Work out the finished part from the listing and answer in its coordinate system (mm). A direction names the side the tool comes from. Round coordinates to 2 decimals unless told otherwise and drop trailing zeros. Order: outer loops, then holes, each group sorted by start corner. A loop starts at its lowest first (then second) coordinate and runs counter-clockwise, first axis right, second up. Notation, with made-up numbers: (-30, 27.25) -> (-23, 27.25) arc R30 cw to (-23, 60.25) -> close; hole circle Ø7 at (14, 4). An arc over 180 degrees is marked (long way). Use one line per item in the form item = value.
```python
from build123d import *

# Parameters (mm, degrees)
F1_DEPTH = 60
F3_DEPTH = 80
F4_W     = 6.1120763421
F4_H     = 50.4245881457
F5_DEPTH = 57.3
F7_DEPTH = 45.7
F8_R     = 30


with BuildPart() as f1:
    # F0 (on Right) → F1 (new body)
    with BuildSketch(Plane.YZ):
        Polygon((-85.0046053529, 28.4824129194), (-95.0890108943, 3.9917188697), (-95.0890108943, -38.8669967651), (43.5715354979, -38.8669967651), (54.0160946548, -6.812999025), (28.4449271858, 52.252791822), (-15.8544126898, 52.252791822), (-15.8544126898, 8.3136055619), (-23.7778741866, 28.4824129194), align=None)
    extrude(amount=F1_DEPTH)

    # F2 (on face) → F3 (join)
    with BuildSketch(Plane.YZ.offset(60)):
        Polygon((-9.2091018375, -8.6017280287), (-15.8544126898, 8.3136055619), (-23.7778741866, 28.4824129194), (-85.0046053529, 28.4824129194), (-95.0890108943, 3.9917188697), (-95.0890108943, -38.8669967651), (43.5715354979, -38.8669967651), (53.433250479, -8.6017280287), align=None)
    extrude(amount=F3_DEPTH)

    # F4 (on face) → F5 (join)
    with BuildSketch(Plane.XY.offset(-8.6017280287)):
        with Locations((78.1879983842, 23.0138575425)):
            Rectangle(F4_W, F4_H)
        with Locations((106.4563281834, 23.0138575425)):
            Rectangle(F4_W, F4_H)
    extrude(amount=F5_DEPTH)

    # F6 (on face) → F7 (cut)
    with BuildSketch(Plane.YZ.offset(109.5123663545)):
        Polygon((-2.1984365303, 48.6982719713), (-2.1984365303, 32.272413373), (24.9238815159, 32.272413373), (48.2261516154, 7.0601203479), (48.2261516154, 48.6982719713), align=None)
    extrude(amount=-F7_DEPTH, mode=Mode.SUBTRACT)

    # F8
    f8_edges = [f1.edges().sort_by_distance(p)[0] for p in [
        (106.456328, 48.226152, 7.06012),
        (106.456328, 24.923882, 32.272413),
        (78.187998, 24.923882, 32.272413),
        (78.187998, 48.226152, 7.06012),
    ]]
    fillet(f8_edges, radius=F8_R)


solid = f1.part
```
Item 1: The part is cut by section B-B, the plane x = 94. Give the vertices of the cut face in (y, z).
Findings:
outline = (-95.09, -38.87) -> (43.57, -38.87) -> (53.43, -8.6) -> (-9.21, -8.6) -> (-23.78, 28.48) -> (-85, 28.48) -> (-95.09, 3.99) -> close
Item 2: The part is cut by section A-A, the plane z = 18. Give the vertices of the cut face in (x, y).
Findings:
outline = (0, -89.32) -> (140, -89.32) -> (140, -19.66) -> (0, -19.66) -> close; (0, -15.85) -> (60, -15.85) -> (60, 43.27) -> (0, 43.27) -> close; (75.13, -2.2) -> (81.24, -2.2) -> (81.24, 38.12) -> (75.13, 38.12) -> close; (103.4, -2.2) -> (109.51, -2.2) -> (109.51, 38.12) -> (103.4, 38.12) -> close
Item 3: Consider line 1 along X through (y, z) = (18, 6); line 2 along Y through (x, z) = (13, 20.5); line 3 along Z through (x, y) = (109, 6). Determine where each line is inside the solid, lowest interval first.
Findings:
line_1 = 0 to 60, 75.13 to 81.24, 103.4 to 109.51
line_2 = -88.29 to -20.64, -15.85 to 42.19
line_3 = -38.87 to 32.27
Item 4: The part is cut by section C-C, the plane y = -59.5. Give the vertices of the cut face in (x, z), and give its area (3 significant figures).
Findings:
outline = (0, -38.87) -> (140, -38.87) -> (140, 28.48) -> (0, 28.48) -> close
area = 9,430 mm^2
Item 5: The part is cut by section D-D, the plane x = 55. Give the vertices of the cut face in (y, z), and give its area (3 significant figures).
Findings:
outline = (-95.09, -38.87) -> (43.57, -38.87) -> (54.02, -6.81) -> (28.44, 52.25) -> (-15.85, 52.25) -> (-15.85, 8.31) -> (-23.78, 28.48) -> (-85, 28.48) -> (-95.09, 3.99) -> close
area = 10,600 mm^2
Item 6: For faces 1 (the flat face through (106.499, 36.999, 19.207)), 2 (the flat face through (30, -15.854, 31)), 3 (the flat face through (69, -54, 28.482)), 4 (the flat face through (60, 11, 22)), 5 (the flat face through (106, 5, 32.272)), determine the directions among +Z, -Z, +X, -X, +Y, -Y from which every point of the face is accessible in a straight line to the end or side of a thin tool.
Findings:
face_1 = +Z, +X, +Y
face_2 = +Z, +X, -X
face_3 = +Z, +X, -X, -Y
face_4 = +Z, +Y
face_5 = +Z, +X, +Y, -Y
Item 7: Determine the mould class of faces 6 (the flat face through (106, -2.198, 12)), 7 (the flat face through (69.02, 48.721, -23.064)), 8 (the flat face through (109.512, 23, 12)) for opening direction Y: released by +Y, released by -Y, zero draft, split by the parting line, or undercut.
Findings:
face_6 = undercut
face_7 = released by +Y
face_8 = zero draft
Item 8: Flat-ended cylindrical pins translate along their axes: P1, Ø1.8, axis at x = 106, y = 4, coming from the +Z side; P2, Ø6.5, axis at x = 79, z = 13, coming from the -Y side; P3, Ø2, axis at x = 79.5, z = -7, coming from the +Y side. Find the tip coordinate at first contact, or state that the pin passes through.
Findings:
P1 = 32.27
P2 = -92.72
P3 = 48.23
